Geometry: see drawing. Coordinates: mm, zero at the bounding-box minimum. A direction names the side the tool comes from. Coordinates: 2 decimals unless noted, no trailing zeros. Loops run counter-clockwise (first coordinate to the right, second up) from the corner with the lowest first, then second, coordinate; pieces in that order, holes last.
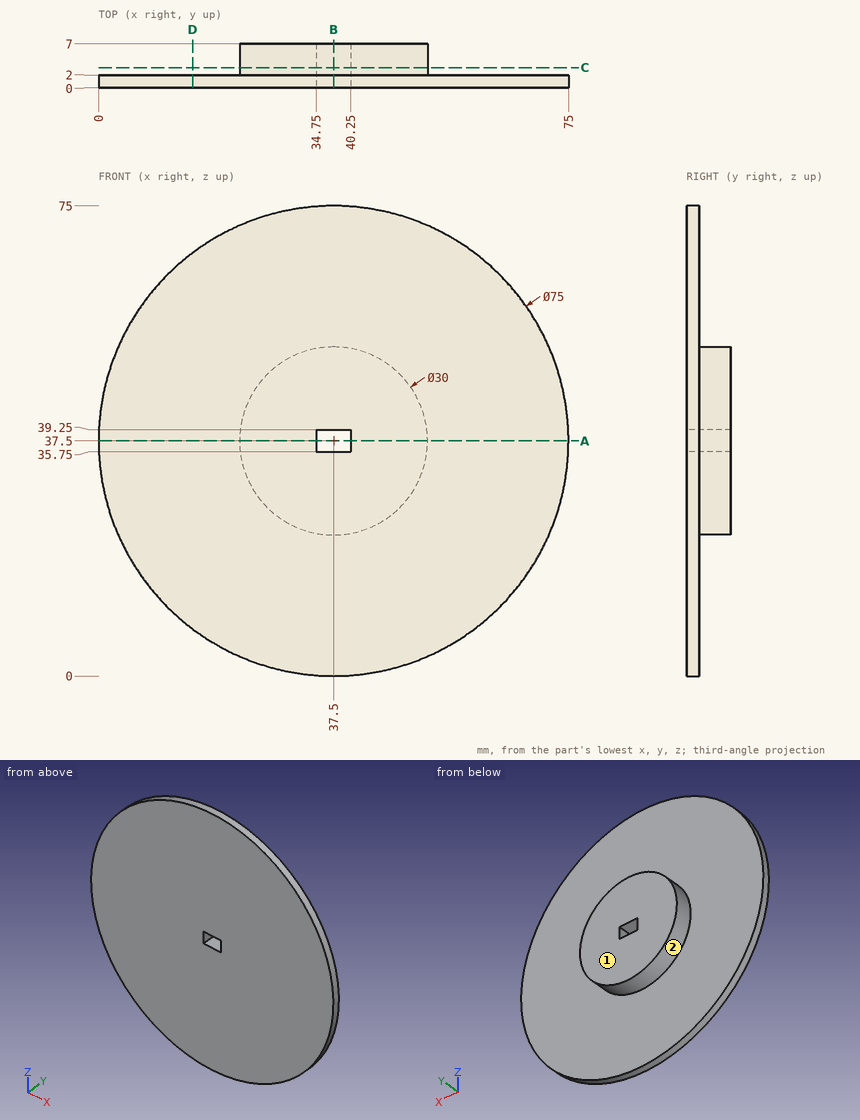
Item 1: Section query C-C (y = 3.25). Output: boundary loops of the cut face in (x, z).
Result:
outline: circle Ø30 at (37.5, 37.5); hole (34.75, 35.75) - (40.25, 35.75) - (40.25, 39.25) - (34.75, 39.25) - close
Item 2: Line query: L1, parallel to X at y = 4.75, z = 37.5; L2, parallel to Y at x = 62.5, z = 53.5; L3, parallel to X at y = 4.75, z = 36. Output: solid intervals per line, ascending.
Result:
L1: x = 22.5 to 34.75, 40.25 to 52.5
L2: y = 0 to 2
L3: x = 22.58 to 34.75, 40.25 to 52.42
Item 3: Reachability of the marked faces 1 and 2 from +Z, -Z, +X, -X, +Y, -Y: full face, straight path, thin tool, end or side. Return the list, or none.
Result:
face 1: +Z, -Z, +X, -X, +Y
face 2: +Y
Item 4: Contact query for flat-ended pins moving along their axis: P1, Ø1.5, axis at y = 3, z = 19.5, coming from the -X side; P2, Ø5, axis at x = 59, z = 50, coming from the +Y side; P3, Ø3, axis at x = 51, y = 2.5, coming from the -Z side; P4, Ø3, axis at y = 4, z = 38, coming from the +X side. Output: stop coordinate, or through.
Result:
P1: passes through
P2: stops at y = 2
P3: stops at z = 2
P4: stops at x = 52.5
Item 5: Section query A-A (z = 37.5). Output: boundary loops of the cut face in (x, y).
Result:
outline: (0, 0) - (34.75, 0) - (34.75, 7) - (22.5, 7) - (22.5, 2) - (0, 2) - close; (40.25, 0) - (75, 0) - (75, 2) - (52.5, 2) - (52.5, 7) - (40.25, 7) - close
Item 6: Section query D-D (x = 15). Output: boundary loops of the cut face in (y, z), then the cut area to 3 significant figures.
Result:
outline: (0, 7.5) - (2, 7.5) - (2, 67.5) - (0, 67.5) - close
area: 120 mm2
Item 7: Section query B-B (x = 37.5). Output: boundary loops of the cut face in (y, z).
Result:
outline: (0, 0) - (2, 0) - (2, 22.5) - (7, 22.5) - (7, 35.75) - (0, 35.75) - close; (0, 39.25) - (7, 39.25) - (7, 52.5) - (2, 52.5) - (2, 75) - (0, 75) - close
